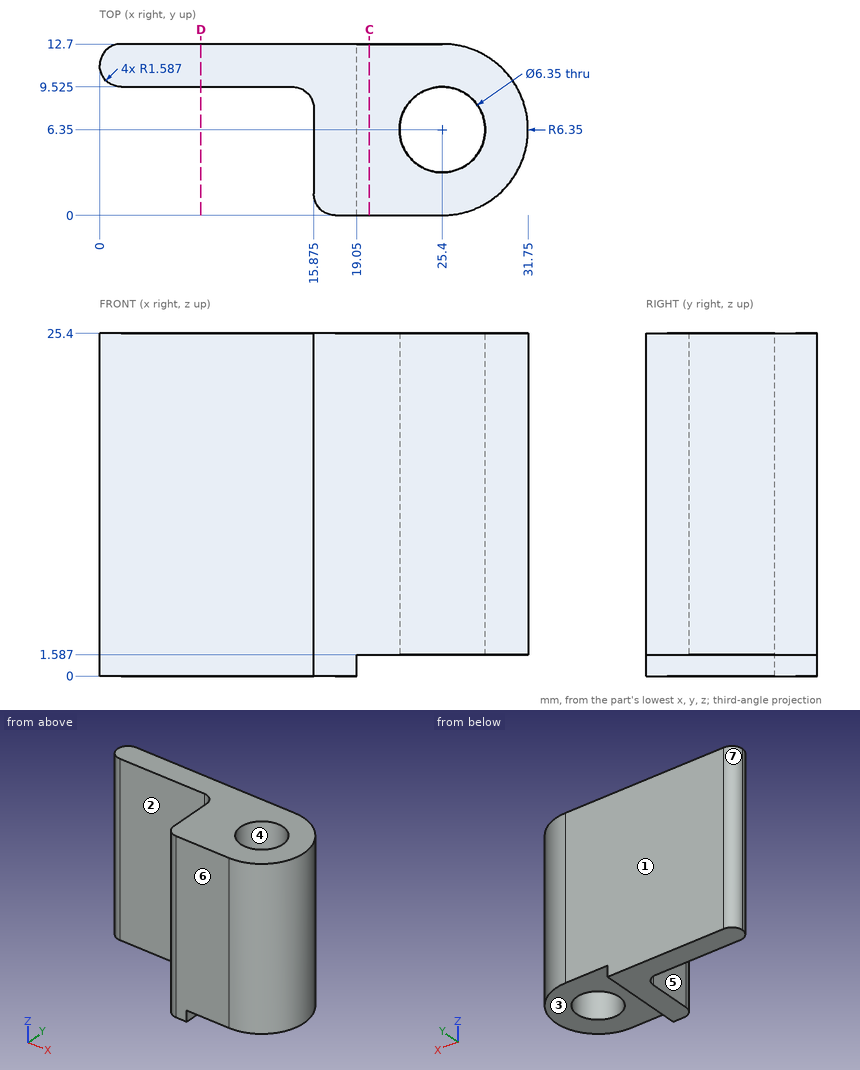
Answer from the drawing. Dimensions are ordinates in mm from the lowest x, y and z of the part. A direction names the side the tool comes from. Round coordinates to 2 decimals unless told otherwise and drop trailing zeros. Loops run counter-clockwise (first coordinate to the right, second up) from the corner with the lowest first, then second, coordinate; pieces in that order, holes last. Notation, with made-up numbers: (58, 23) - (88, 23) arc R26 ccw to (88, 47) - close; hole circle Ø7 at (-29.75, -10.75). An arc over 180 degrees is marked (long way). One line per item, written item: value.
Q1. Each of these flat-tipped pins is pushed along its axis until it touches: pin 1 Ø1 at (x, y) = (6, 11) entering from -Z; pin 2 Ø6.5 at (x, y) = (22.5, 3.5) entering from -Z; pin 3 Ø1.7 at (y, z) = (4, 0.5) entering from +X; pin 4 Ø2 at (y, z) = (1.5, 22.5) entering from +X. Where does it stop, or does it pass through?
Check values:
pin 1: z = 0
pin 2: z = 1.59
pin 3: x = 19.05
pin 4: x = 30.45
Q2. Find section D-D on x = 7.5. Give the vertices of the cut face in (y, z) (1 decimal).
Check values:
outline: (9.5, 0) - (12.7, 0) - (12.7, 25.4) - (9.5, 25.4) - close
Q3. The mould has two halves that part along Y. Classify the marked faces 4, 5, 6 and 7: +Y half, -Y half, draft (parallel to the pull), parting line (faces both ways), or undercut.
Check values:
face 4: undercut
face 5: draft
face 6: -Y half
face 7: +Y half
Q4. Find section C-C on x = 20. Give the vertices of the cut face in (y, z), and give its area (3 significant figures).
Check values:
outline: (0, 1.59) - (12.7, 1.59) - (12.7, 25.4) - (0, 25.4) - close
area: 302 mm2
Q5. Straight lines are drawn through the part: probe 1 along Y at (x, z) = (25.4, 15.75) (1 decimal); probe 2 along X at (y, z) = (6.5, 21) (1 decimal); probe 3 along Z at (x, y) = (26, 1). For each, find the intervals that lie inside material, in ascending order.
Check values:
probe 1: 0 to 3.2, 9.5 to 12.7
probe 2: 15.9 to 22.2, 28.6 to 31.7
probe 3: 1.59 to 25.4
Q6. For the marked faces 1, 2 and 3, determine the directions among +Z, -Z, +X, -X, +Y, -Y from which every point of the face is accessible in a straight line to the end or side of a thin tool.
Check values:
face 1: +Z, -Z, +X, -X, +Y
face 2: +Z, -Z, -X, -Y
face 3: -Z, +X, +Y, -Y
